Model file for the job. Use its own axes, mm. A direction names the side the tool comes from. Coordinates: 2 decimals unless noted, no trailing zeros. Order: outer loops, then holes, each group sorted by start corner. A loop starts at its lowest first (then second) coordinate and runs counter-clockwise, first axis right, second up. Notation, with made-up numbers: M -16,23.5 L 21,23.5 A22 cw 21,55.5 Z; hole C 13,21 d3. An arc over 180 degrees is marked long. Return JSON: item names as keys, results as strings.
```python
from build123d import *

# Parameters (mm, degrees)
F1_DEPTH = 50.8
F2_R     = 19.05
F3_R     = 1.27
F4_W     = 30.48
F4_H     = 45.66285
F5_DEPTH = 19.05
F7_D     = 3.2512
F8_R     = 0.3175


with BuildPart() as f1:
    # F0 (on Front) → F1 (new body)
    with BuildSketch(Plane.XZ):
        Polygon((0, 38.1), (0, 0), (101.6, 0), (73.369475, 19.463853), (30.235227, 30.198802), (20.174297, 28.783426), (9.532238, 24.613116), align=None)
    extrude(amount=F1_DEPTH)

    # F2
    f2_edges = [f1.edges().sort_by_distance(p)[0] for p in [
        (30.235227, -25.4, 30.198802),
        (73.369475, -25.4, 19.463853),
        (20.174297, -25.4, 28.783426),
    ]]
    fillet(f2_edges, radius=F2_R)

    # F3
    f3_edges = [f1.edges().sort_by_distance(p)[0] for p in [
        (101.6, -25.4, 0),
    ]]
    fillet(f3_edges, radius=F3_R)

    # F4 (on face) → F5 (cut)
    with BuildSketch(Plane(origin=(8.84079, 0, 35.5233), x_dir=(0.970399, 0, -0.241506), z_dir=(0.241506, 0, 0.970399))):
        with Locations((44.906641, -25.403175)):
            Rectangle(F4_W, F4_H)
    extrude(amount=-F5_DEPTH, mode=Mode.SUBTRACT)

    # F7 (through all)
    with Locations(Plane.XZ.offset(50.8)):
        with Locations((12.7, 3.429), (86.033185, 3.429)):
            Hole(F7_D / 2)

    # F8
    f8_edges = [f1.edges().sort_by_distance(p)[0] for p in [
        (0, -25.4, 38.1),
    ]]
    fillet(f8_edges, radius=F8_R)


solid = f1.part
```
Item 1: Wall check: line 1 (Z direction, x = 29.5, y = -5); line 2 (Y direction, x = 59, z = 14.5); line 3 (X direction, y = -34, z = 15.5). Give the ranges that are in metal, low to high.
Check result:
{"line 1": "z = 0 to 29.87", "line 2": "y = -50.8 to -48.23, -2.57 to 0", "line 3": "x = 0 to 34.43, 65.84 to 79.12"}
Item 2: 3-axis set-ups, long thin cutter, end or side, ignore diameter. For faces 5 (the flat face through (64.94, -25.72, 11.88)), 6 (the flat face through (13.872, -25.044, 26.314)), 7 (the flat face through (0, -25, 19)): which of +Z, -Z, +X, -X, +Y, -Y reach the whole face in a straight line?
Check result:
{"face 5": "+Z", "face 6": "+Z, +Y, -Y", "face 7": "+Z, -Z, -X, +Y, -Y"}
Item 3: Saw through at D-D (z = 22). Write the cut outline in (x, y), and give its area (3 significant figures).
Check result:
{"outline": "M 0,-50.8 L 63.18,-50.8 L 63.18,-48.23 L 36.05,-48.23 L 36.05,-2.57 L 63.18,-2.57 L 63.18,0 L 0,0 Z", "area": "1,970 mm2"}
Item 4: Saw through at B-B (x = 12.7). Write the cut outline in (y, z), and give its area (3 significant figures).
Check result:
{"outline": "M -50.8,0 L 0,0 L 0,1.8 L -50.8,1.8 Z; M -50.8,5.05 L 0,5.05 L 0,25.85 L -50.8,25.85 Z", "area": "1,150 mm2"}
Item 5: Saw through at C-C (y = -8). Count the separate pieces of the cut face and the enclosed holes in it, and give its area (3 significant figures).
Check result:
{"separate pieces": "1", "enclosed holes": "2", "area": "1,620 mm2"}
Item 6: Saw through at A-A (z = 12). Write the cut outline in (x, y), and give its area (3 significant figures).
Check result:
{"outline": "M 0,-50.8 L 84.2,-50.8 L 84.2,0 L 0,0 Z; hole M 33.56,-48.23 L 64.97,-48.23 L 64.97,-2.57 L 33.56,-2.57 Z", "area": "2,840 mm2"}
Item 7: Pull direction Z, two halves, no side cores. Call faces 1 (the cylindrical face through (87.323, -25.044, 2.44)), 2 (the flat face through (37.26, -30.93, 28.45)), 3 (the flat face through (35.36, -25.72, 19.24)), 4 (the cylindrical face through (98.74, -25.76, 0.91)): +Z half, -Z half, draft (parallel to the pull), parting line (faces both ways), or undercut.
Check result:
{"face 1": "undercut", "face 2": "+Z half", "face 3": "undercut", "face 4": "parting line"}
Item 8: Drop flat-ended pins along their axis: pin 1 Ø12 at (y, z) = (-26, 15.5) entering from +X; pin 2 Ø2.5 at (x, z) = (12.7, 3.429) entering from +Y; pin 3 Ø12 at (x, y) = (32.5, -18.5) entering from +Z; pin 4 Ø3 at (x, y) = (54.5, -17.5) entering from +Z. Give the stop position or say it passes through.
Check result:
{"pin 1": "stops at x = 87.82", "pin 2": "passes through", "pin 3": "stops at z = 29.87", "pin 4": "stops at z = 4.9"}
